Here's how the part is built. I have some questions about the finished solid (model axes, mm). Face numbers are marked on the shaded views. A direction names the side the tool comes from. Coordinates: 2 decimals unless noted, no trailing zeros. Write each loop counter-clockwise with the first axis right and the second up, starting at its lowest first coordinate (ties: lowest second). Pieces come first, ordered by that corner, then holes.
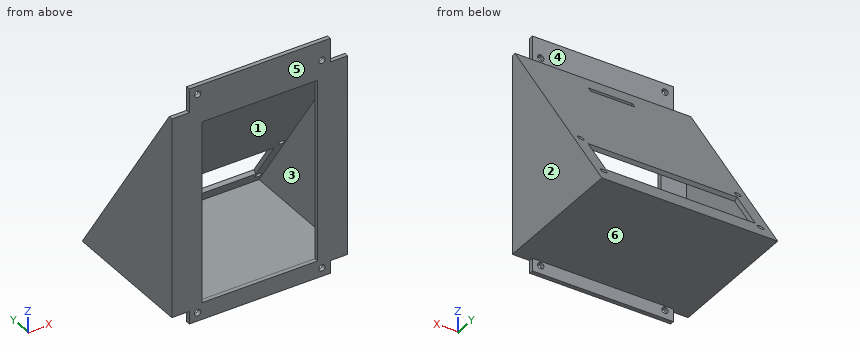
```python
from build123d import *

# Parameters (mm, degrees)
SKETCH1_W           = 67.34
SKETCH1_H           = 113.06
SKETCH1_R           = 1.5
SKETCH1_W_2         = 55.34
SKETCH1_H_2         = 101.06
BOSS_EXTRUDE1_DEPTH = 2
BOSS_EXTRUDE2_DEPTH = 42
SKETCH4_W           = 55.34
SKETCH4_H           = 2
BOSS_EXTRUDE5_DEPTH = 11.970099
CUT_EXTRUDE1_REACH  = 60.174
SKETCH5_R           = 1.5
SKETCH5_W           = 71.2
SKETCH5_H           = 24.2
SKETCH5_W_2         = 21
SKETCH5_H_2         = 3
BOSS_EXTRUDE6_DEPTH = 2
SKETCH7_W           = 8.33
SKETCH7_H           = 95.603562999
BOSS_EXTRUDE7_DEPTH = 2
SKETCH8_W           = 55.34
SKETCH8_H           = 2
BOSS_EXTRUDE8_DEPTH = 2.076588


with BuildPart() as part:
    # Sketch1 → Boss-Extrude1 (new body)
    with BuildSketch(Plane(origin=(0, 0, 0), x_dir=(1, 0, 0), z_dir=(0, 1, 0))):
        with Locations((-64.664649644, -123.030692549)):
            Rectangle(SKETCH1_W, SKETCH1_H)
        with Locations((-34.994649644, -70.500692549)):
            Circle(SKETCH1_R, mode=Mode.SUBTRACT)
        with Locations((-94.334649644, -70.500692549)):
            Circle(SKETCH1_R, mode=Mode.SUBTRACT)
        with Locations((-94.334649644, -175.560692549)):
            Circle(SKETCH1_R, mode=Mode.SUBTRACT)
        with Locations((-34.994649644, -170.434906111)):
            Circle(SKETCH1_R, mode=Mode.SUBTRACT)
        with Locations((-64.664649644, -123.030692549)):
            Rectangle(SKETCH1_W_2, SKETCH1_H_2, mode=Mode.SUBTRACT)
    extrude(amount=BOSS_EXTRUDE1_DEPTH)

    # Sketch3 → Boss-Extrude2 (add, symmetric)
    with BuildSketch(Plane(origin=(-64.664649644, 0, 0), x_dir=(0, 0, -1), z_dir=(1, 0, 0))):
        Polygon((-161.590593962, 4), (-161.590593962, 2), (-168.180843703, 2), (-72.577280704, 65.913681963), (-72.577280704, 2), (-74.577280704, 2), (-74.577280704, 4), (-74.577280704, 62.1708574), align=None)
    extrude(amount=BOSS_EXTRUDE2_DEPTH, both=True)

    # Sketch4 → Boss-Extrude5 (add)
    with BuildSketch(Plane(origin=(0, 0, 173.560692549), x_dir=(-1, 0, 0), z_dir=(0, 0, -1))):
        with Locations((64.664649644, 1)):
            Rectangle(SKETCH4_W, SKETCH4_H)
    extrude(amount=BOSS_EXTRUDE5_DEPTH)

    # Sketch5 → Cut-Extrude1 (cut, up to next)
    with BuildSketch(Plane(origin=(0, 79.087200487, 52.872027158), x_dir=(1, 0, 0), z_dir=(0, 0.83133533, 0.555771148)), mode=Mode.PRIVATE) as cut_extrude1_sk1:
        with Locations((-26.824649644, -33.033134975)):
            Circle(SKETCH5_R)
    cut_extrude1_tool1 = extrude(cut_extrude1_sk1.sketch, amount=-CUT_EXTRUDE1_REACH, mode=Mode.PRIVATE) & part.part
    add(cut_extrude1_tool1.solids().sort_by_distance((-26.82465, 60.728337, 80.333639))[0], mode=Mode.SUBTRACT)
    # Sketch5 → Cut-Extrude1 (cut, up to next)
    with BuildSketch(Plane(origin=(0, 79.087200487, 52.872027158), x_dir=(1, 0, 0), z_dir=(0, 0.83133533, 0.555771148)), mode=Mode.PRIVATE) as cut_extrude1_sk2:
        with Locations((-26.824649644, -63.403134975)):
            Circle(SKETCH5_R)
    cut_extrude1_tool2 = extrude(cut_extrude1_sk2.sketch, amount=-CUT_EXTRUDE1_REACH, mode=Mode.PRIVATE) & part.part
    add(cut_extrude1_tool2.solids().sort_by_distance((-26.82465, 43.849567, 105.581293))[0], mode=Mode.SUBTRACT)
    # Sketch5 → Cut-Extrude1 (cut, up to next)
    with BuildSketch(Plane(origin=(0, 79.087200487, 52.872027158), x_dir=(1, 0, 0), z_dir=(0, 0.83133533, 0.555771148)), mode=Mode.PRIVATE) as cut_extrude1_sk3:
        with Locations((-101.824649644, -63.403134975)):
            Circle(SKETCH5_R)
    cut_extrude1_tool3 = extrude(cut_extrude1_sk3.sketch, amount=-CUT_EXTRUDE1_REACH, mode=Mode.PRIVATE) & part.part
    add(cut_extrude1_tool3.solids().sort_by_distance((-101.82465, 43.849567, 105.581293))[0], mode=Mode.SUBTRACT)
    # Sketch5 → Cut-Extrude1 (cut, up to next)
    with BuildSketch(Plane(origin=(0, 79.087200487, 52.872027158), x_dir=(1, 0, 0), z_dir=(0, 0.83133533, 0.555771148)), mode=Mode.PRIVATE) as cut_extrude1_sk4:
        with Locations((-101.824649644, -33.033134975)):
            Circle(SKETCH5_R)
    cut_extrude1_tool4 = extrude(cut_extrude1_sk4.sketch, amount=-CUT_EXTRUDE1_REACH, mode=Mode.PRIVATE) & part.part
    add(cut_extrude1_tool4.solids().sort_by_distance((-101.82465, 60.728337, 80.333639))[0], mode=Mode.SUBTRACT)
    # Sketch5 → Cut-Extrude1 (cut, up to next)
    with BuildSketch(Plane(origin=(0, 79.087200487, 52.872027158), x_dir=(1, 0, 0), z_dir=(0, 0.83133533, 0.555771148)), mode=Mode.PRIVATE) as cut_extrude1_sk5:
        with Locations((-64.664649644, -47.803134975)):
            Rectangle(SKETCH5_W, SKETCH5_H)
    cut_extrude1_tool5 = extrude(cut_extrude1_sk5.sketch, amount=-CUT_EXTRUDE1_REACH, mode=Mode.PRIVATE) & part.part
    add(cut_extrude1_tool5.solids().sort_by_distance((-64.66465, 52.519597, 92.612462))[0], mode=Mode.SUBTRACT)
    # Sketch5 → Cut-Extrude1 (cut, up to next)
    with BuildSketch(Plane(origin=(0, 79.087200487, 52.872027158), x_dir=(1, 0, 0), z_dir=(0, 0.83133533, 0.555771148)), mode=Mode.PRIVATE) as cut_extrude1_sk6:
        with Locations((-64.664649644, -127.203134975)):
            Rectangle(SKETCH5_W_2, SKETCH5_H_2)
    cut_extrude1_tool6 = extrude(cut_extrude1_sk6.sketch, amount=-CUT_EXTRUDE1_REACH, mode=Mode.PRIVATE) & part.part
    add(cut_extrude1_tool6.solids().sort_by_distance((-64.66465, 8.391368, 158.620487))[0], mode=Mode.SUBTRACT)

    # Sketch6 → Boss-Extrude6 (add)
    with BuildSketch(Plane(origin=(-22.664649644, 0, 0), x_dir=(0, 0, -1), z_dir=(1, 0, 0))):
        Polygon((-168.180843703, 2), (-168.180843703, 0), (-72.577280704, 0), (-72.577280704, 2), (-72.577280704, 65.913681963), align=None)
    boss_extrude6 = extrude(amount=-BOSS_EXTRUDE6_DEPTH)

    # Sketch7 → Boss-Extrude7 (add)
    with BuildSketch(Plane.XZ.offset(-2)):
        with Locations((-28.829649644, 120.379062204)):
            Rectangle(SKETCH7_W, SKETCH7_H)
    boss_extrude7 = extrude(amount=BOSS_EXTRUDE7_DEPTH)

    # Mirror1: Boss-Extrude6, Boss-Extrude7 across plane
    add(boss_extrude6.mirror(Plane(origin=(-64.664649644, 0, 0), x_dir=(0, 0, 1), z_dir=(1, 0, 0))))
    add(boss_extrude7.mirror(Plane(origin=(-64.664649644, 0, 0), x_dir=(0, 0, 1), z_dir=(1, 0, 0))))

    # Sketch8 → Boss-Extrude8 (add)
    with BuildSketch(Plane.XY.offset(72.500692549)):
        with Locations((-64.664649644, 1)):
            Rectangle(SKETCH8_W, SKETCH8_H)
    extrude(amount=BOSS_EXTRUDE8_DEPTH)


solid = part.part
```
1) On a 3-axis mill with a long thin cutter (end or side, diameter ignored), from which of +Z, -Z, +X, -X, +Y, -Y can I reach the whole of each face in a straight line? I mean the marked faces 1 and 2. Say none if no direction works.
Values follow:
face 1: none
face 2: +Z, -Z, +X, +Y, -Y
2) Imagine slicing it at B-B on x = -63.5. Please give me the cut outline in (y, z), then the cut area to 3 significant figures.
Values follow:
outline: (0, 66.5) - (2, 66.5) - (2, 72.58) - (65.91, 72.58) - (59.24, 82.55) - (57.58, 81.44) - (62.17, 74.58) - (0, 74.58) - close; (0, 161.59) - (4, 161.59) - (5.9, 158.76) - (7.56, 159.87) - (2, 168.18) - (2, 179.56) - (0, 179.56) - close; (7.56, 156.26) - (44.13, 101.56) - (45.79, 102.67) - (9.23, 157.37) - close
area: 348 mm2
3) We'd pull the mould along Y, two halves only. Please class the marked faces 3, 4, 5 and 6: pulls with the +Y half, pulls with the -Y half, needs draft (parallel to the pull), parting line crosses it, or undercut.
Values follow:
face 3: undercut
face 4: pulls with the +Y half
face 5: pulls with the -Y half
face 6: needs draft
4) Will these pins go through, and if not, where does the flat tip stop? pin 1 (5 mm diameter, centred on x = -94.33, z = 70.5, fed in from +Y); pin 2 (0.6 mm diameter, centred on x = -53.5, y = 3, fed in from -Z); pin 3 (1.5 mm diameter, centred on x = -86.5, y = 29.5, fed in from +Z); pin 4 (6 mm diameter, centred on y = 7.5, z = 166.5, fed in from -X).
Values follow:
pin 1: stops at y = 65.91
pin 2: stops at z = 72.58
pin 3: stops at z = 128.17
pin 4: passes through
5) I need wall thicknesses on probe 1 along X at (y, z) = (24, 110); probe 2 along Z at (x, y) = (-71.5, 43); probe 3 along Z at (x, y) = (-99.5, 5). Which ranges of each line are inside material? Lowest first, please.
Values follow:
probe 1: x = -106.66 to -104.66, -24.66 to -22.66
probe 2: z = 72.58 to 74.58, 103.25 to 106.85
probe 3: z = 72.58 to 74.58, 160.09 to 163.69
6) Imagine slicing it at A-A on x = -77.5. Please give me the cut outline in (y, z), then the cut area to 3 significant figures.
Values follow:
outline: (0, 66.5) - (2, 66.5) - (2, 72.58) - (65.91, 72.58) - (59.24, 82.55) - (57.58, 81.44) - (62.17, 74.58) - (0, 74.58) - close; (0, 161.59) - (4, 161.59) - (44.13, 101.56) - (45.79, 102.67) - (2, 168.18) - (2, 179.56) - (0, 179.56) - close
area: 354 mm2
7) Imagine slicing it at C-C on y = 18.5. Please give me the cut outline in (x, z), then the cut area to 3 significant figures.
Values follow:
outline: (-106.66, 72.58) - (-22.66, 72.58) - (-22.66, 143.5) - (-106.66, 143.5) - close; hole (-104.66, 74.58) - (-24.66, 74.58) - (-24.66, 139.9) - (-104.66, 139.9) - close
area: 732 mm2
8) Imagine slicing it at D-D on z = 97. Please give me the cut outline in (x, y), then the cut area to 3 significant figures.
Values follow:
outline: (-106.66, 0) - (-92.33, 0) - (-92.33, 2) - (-104.66, 2) - (-104.66, 47.18) - (-100.26, 47.18) - (-100.26, 49.59) - (-106.66, 49.59) - close; (-36.99, 0) - (-22.66, 0) - (-22.66, 49.59) - (-29.06, 49.59) - (-29.06, 47.18) - (-24.66, 47.18) - (-24.66, 2) - (-36.99, 2) - close
area: 269 mm2
